Here's how the part is built. I have some questions about the finished solid (model axes, mm). A direction names the side the tool comes from. Coordinates: 2 decimals unless noted, no trailing zeros. Loops run counter-clockwise (first coordinate to the right, second up) from the corner with the lowest first, then second, coordinate; pieces in that order, holes last. Notation, with made-up numbers: M 18,78 L 29,78 A22 cw 29,111 Z; hole C 18.25,38 d10. An arc over 180 degrees is marked long. Use CSV: the item, a comma, the result in double quotes. Start each with the question number.
Q1. If we section it at C-C (x = -21): State how many separate pieces and enclosed holes the cut face has, and give its area (3 significant figures).
Q2. Please list where these lines run through material, in increasing order: probe 1 along Y at (x, z) = (0, 0); probe 2 along X at (y, z) = (11, 1.5); probe 3 along X at (y, z) = (1, -33). Write a range as [from, to].
Q3. For pin 1 Ø6 at (x, z) = (2, -2.5) entering from +Y; pin 2 Ø1.9 at (x, y) = (1, 0.5) entering from -Z; pin 3 Ø3 at (y, z) = (4.5, -1) entering from +X; pin 4 Ø6 at (x, y) = (-0.5, 2.5) entering from -Z, each with a flat end and sliding along its axis, tell me the tip position at first contact or that it passes through.
Q4. If we mould it in two halves opening along Z, with no side actions, what happens to faces 1 (the cylindrical face through (0, 25, 1)), 2 (the flat face through (0, 0, -16)), 3 (the flat face through (0, 0, 3)), 4 (the flat face through (-3, 5, -18))? For each: +Z half, -Z half, draft (parallel to the pull), parting line (faces both ways), or undercut.
Q5. Which directions (+Z, -Z, +X, -X, +Y, -Y) give clear straight access to the entire face, cutting with the end or side of a thin tool? Please do faces 5 (the cylindrical face through (-5.54, 2.3, -27.38)), 6 (the flat face through (3, 5, -19)), 7 (the cylindrical face through (0, -20, 1)).
Q6. If we section it at A-A (z = -24.5): Please give me the cut outline in (x, y).
from build123d import *

# Parameters (mm, degrees)
SKETCH_2_R               = 6.5
CUT_EXTRUDE_1_DEPTH      = 28
CHAMFER_1_SIZE           = 0.5
SKETCH_3_R               = 2.5
CUT_EXTRUDE_2_DEPTH      = 23
SKETCH_4_R               = 3.1
CUT_EXTRUDE_3_DEPTH      = 20
SKETCH_5_R               = 16.017465931
CUT_EXTRUDE_4_DEPTH      = 30.8
SKETCH_6_R               = 12
SKETCH_6_R_2             = 9
EXTRUDE_1_DEPTH          = 13
SKETCH_7_R               = 12
SKETCH_7_R_2             = 9
CUT_EXTRUDE_5_DEPTH      = 0.5
CHAMFER_2_SIZE           = 0.5
CUT_EXTRUDE_6_DEPTH      = 20.5
CUT_EXTRUDE_6_DEPTH_BACK = 30.5
SKETCH_8_R               = 1.4


with BuildPart() as part:
    # 草图1 → 旋转1 (revolve)
    with BuildSketch(Plane(origin=(0, 0, 0), x_dir=(1, 0, 0), z_dir=(0, 1, 0))):
        Polygon((-6, 20.000076755), (-6, 36.000076755), (0, 36.000076755), (0, 30.000076755), (0, -33.8), (-9.249924022, -33.8), (-9.75, -33.299919915), (-9.75, -3), (-27.5, -3), (-27.5, 1.000001333), (-27.000001277, 1.5), (-9, 1.5), (-9, 6.5), (-9, 13.000076755), (-6, 13.000076755), (-6, 18.000076755), (-5.5, 18.000076755), (-5.5, 19.000076755), (-6, 19.000076755), align=None)
    revolve(axis=Axis((0, 0, -30.000076755), (0, 0, 1)))

    # 草图2 → 切除-拉伸1 (cut)
    with BuildSketch(Plane.XY.offset(33.8)):
        Circle(SKETCH_2_R)
    extrude(amount=-CUT_EXTRUDE_1_DEPTH, mode=Mode.SUBTRACT)

    # 倒角1
    chamfer_1_edges = [part.edges().sort_by_distance(p)[0] for p in [
        (-6.5, 0, 33.8),
    ]]
    chamfer(chamfer_1_edges, length=CHAMFER_1_SIZE)

    # 草图3 → 切除-拉伸2 (cut)
    with BuildSketch(Plane(origin=(0, 0, -1.5), x_dir=(-1, 0, 0), z_dir=(0, 0, -1))):
        with Locations((0, 22.5)):
            Circle(SKETCH_3_R)
        with Locations((19.485571585, 11.25)):
            Circle(SKETCH_3_R)
        with Locations((19.485571585, -11.25)):
            Circle(SKETCH_3_R)
        with Locations((0, -22.5)):
            Circle(SKETCH_3_R)
        with Locations((-19.485571585, -11.25)):
            Circle(SKETCH_3_R)
        with Locations((-19.485571585, 11.25)):
            Circle(SKETCH_3_R)
    extrude(amount=-CUT_EXTRUDE_2_DEPTH, mode=Mode.SUBTRACT)

    # 草图4 → 切除-拉伸3 (cut)
    with BuildSketch(Plane(origin=(0, 0, -36.000076755), x_dir=(-1, 0, 0), z_dir=(0, 0, -1))):
        Circle(SKETCH_4_R)
    extrude(amount=-CUT_EXTRUDE_3_DEPTH, mode=Mode.SUBTRACT)

    # 草图5 → 切除-拉伸4 (cut)
    with BuildSketch(Plane.XY.offset(33.8)):
        Circle(SKETCH_5_R)
    extrude(amount=-CUT_EXTRUDE_4_DEPTH, mode=Mode.SUBTRACT)

    # 草图6 → 凸台-拉伸1 (add)
    with BuildSketch(Plane(origin=(0, 0, -13.000076755), x_dir=(-1, 0, 0), z_dir=(0, 0, -1))):
        Circle(SKETCH_6_R)
        Circle(SKETCH_6_R_2, mode=Mode.SUBTRACT)
    extrude(amount=-EXTRUDE_1_DEPTH)

    # 草图7 → 切除-拉伸5 (cut)
    with BuildSketch(Plane(origin=(0, 0, -13.000076755), x_dir=(-1, 0, 0), z_dir=(0, 0, -1))):
        Circle(SKETCH_7_R)
        Circle(SKETCH_7_R_2, mode=Mode.SUBTRACT)
    extrude(amount=-CUT_EXTRUDE_5_DEPTH, mode=Mode.SUBTRACT)

    # 倒角2
    chamfer_2_edges = [part.edges().sort_by_distance(p)[0] for p in [
        (9, 0, -12.500076755),
    ]]
    chamfer(chamfer_2_edges, length=CHAMFER_2_SIZE - 0.0001)  # a hair under: the kernel refuses the full size

    # 草图8 → 切除-拉伸6 (cut, two sides: drawn at the far end of the back side and taken through both)
    with BuildSketch(Plane(origin=(0, 0, 0), x_dir=(1, 0, 0), z_dir=(0, 1, 0)).offset(-CUT_EXTRUDE_6_DEPTH_BACK)):
        with Locations(Location((0, 31.500076755, 0), (0, 0, 90))):
            Circle(SKETCH_8_R)
        with Locations(Location((0, 25.000076755, 0), (0, 0, 90))):
            Circle(SKETCH_8_R)
    extrude(amount=CUT_EXTRUDE_6_DEPTH + CUT_EXTRUDE_6_DEPTH_BACK, mode=Mode.SUBTRACT)


solid = part.part
Results below:
1,separate pieces,"3"
1,enclosed holes,"0"
1,area,"124 mm^2"
2,probe 1,"[-27.5, -25], [-20, 20], [25, 27.5]"
2,probe 2,"[-25.2, -21.97], [-17, 17], [21.97, 25.2]"
2,probe 3,"[-5.92, -2.93], [2.93, 5.92]"
3,pin 1,"y = 27.5"
3,pin 2,"z = -16"
3,pin 3,"x = 27.34"
3,pin 4,"z = -36"
4,face 1,"draft"
4,face 2,"-Z half"
4,face 3,"+Z half"
4,face 4,"undercut"
5,face 5,"-Z"
5,face 6,"none"
5,face 7,"+Z, -Z"
6,outline,"M -1.31,-5.86 L -1.31,-2.81 A3.1 cw -1.31,2.81 L -1.31,5.86 A6 ccw Z; M 1.31,-5.86 A6 ccw 1.31,5.86 L 1.31,2.81 A3.1 cw 1.31,-2.81 Z"
